from build123d import *

# Parameters (mm, degrees)
SKETCH_1_W             = 24
SKETCH_1_H             = 27
EXTRUDE_1_DEPTH        = 10
SKETCH_2_R             = 11
SKETCH_2_R_2           = 4.5
EXTRUDE_2_DEPTH        = 9
CUT_EXTRUDE_START      = -41
SKETCH_3_R             = 4.5
CUT_EXTRUDE_1_DEPTH    = 41
SKETCH_4_R             = 2.1
CUT_EXTRUDE_2_DEPTH    = 37.013519789
CHAMFER_1_SIZE         = 2
HOLE_WIZARD_M4_1_D     = 3.3
HOLE_WIZARD_M4_1_DEPTH = 11.5
HOLE_WIZARD_M4_1_TIP   = 0.991420021


with BuildPart() as part:
    # 草图1 → 凸台-拉伸1 (new body)
    with BuildSketch(Plane.XY):
        Rectangle(SKETCH_1_W, SKETCH_1_H)
    extrude(amount=EXTRUDE_1_DEPTH)

    # 草图2 → 凸台-拉伸2 (add)
    with BuildSketch(Plane.XY):
        Circle(SKETCH_2_R)
        Circle(SKETCH_2_R_2, mode=Mode.SUBTRACT)
    extrude(amount=-EXTRUDE_2_DEPTH)

    # 草图3 → 切除-拉伸1 (cut)
    with BuildSketch(Plane(origin=(0, 0, 0), x_dir=(-1, 0, 0), z_dir=(0, 0, -1)).offset(CUT_EXTRUDE_START)):
        with Locations(Location((0, 0, 0), (0, 0, 180))):
            Circle(SKETCH_3_R)
    extrude(amount=CUT_EXTRUDE_1_DEPTH, mode=Mode.SUBTRACT)

    # 草图4 → 切除-拉伸2 (cut)
    with BuildSketch(Plane(origin=(0, 13.5, 0), x_dir=(1, 0, 0), z_dir=(0, 1, 0))):
        with Locations(Location((-8, -5, 0), (0, 0, 270))):
            Circle(SKETCH_4_R)
        with Locations(Location((8, -5, 0), (0, 0, 270))):
            Circle(SKETCH_4_R)
    extrude(amount=-CUT_EXTRUDE_2_DEPTH, mode=Mode.SUBTRACT)

    # 倒角1
    chamfer_1_edges = [part.edges().sort_by_distance(p)[0] for p in [
        (12, 0, 10),
    ]]
    chamfer(chamfer_1_edges, length=CHAMFER_1_SIZE)

    # M4 螺纹孔1
    with Locations(Plane(origin=(11, 0, 0), x_dir=(0, 0, -1), z_dir=(1, 0, 0))):
        with Locations((3, 0)):
            Hole(HOLE_WIZARD_M4_1_D / 2, depth=HOLE_WIZARD_M4_1_DEPTH)
            with Locations((0, 0, -(HOLE_WIZARD_M4_1_DEPTH + HOLE_WIZARD_M4_1_TIP / 2))):  # 118° drill point
                Cone(0, HOLE_WIZARD_M4_1_D / 2, HOLE_WIZARD_M4_1_TIP, mode=Mode.SUBTRACT)


solid = part.part
Source: CAD feature listing. Evaluate the final solid. Frame: model axes, mm. A direction names the side the tool comes from. Round coordinates to 2 decimals unless told otherwise and drop trailing zeros. Loops run counter-clockwise (first coordinate to the right, second up) from the corner with the lowest first, then second, coordinate; pieces in that order, holes last.
Q1. Section D-D, the plane x = 8. Return loops of the section in (y, z).
Q2. Section C-C, the plane y = 1. Return loops of the section in (x, z).
Q3. Section B-B, the plane x = 0. Return loops of the section in (y, z), plus the area to 3 significant figures.
Q4. Ray query, line 1 (X direction, y = 6, z = 5); line 2 (Z direction, x = 7.5, y = -0.5); line 3 (Z direction, x = 7, y = 0). Return the intervals inside material, ascending.
Q5. First-contact query: P1, Ø3, axis at x = -7.5, z = -7, coming from the -Y side; P2, Ø5.5, axis at y = 0, z = -3, coming from the -X side; P3, Ø4, axis at x = 1.5, z = -5, coming from the +Y side; P4, Ø4, axis at x = -8, z = 5, coming from the -Y side. Flat tips, straight axial feed; report the tip coordinate or a pass-through.
Q6. Section A-A, the plane z = 5. Return loops of the section in (x, y).
Q7. Mould query, pull axis X, two halves, no side actions, for faces 1 (the face through (0, 13.5, 5)), 2 (the face through (11, 0, 9)), 3 (the face through (10.082, 0.189, 4.727)). Classes: pulls with the +X half, pulls with the -X half, needs draft (parallel to the pull), parting line crosses it, or undercut.
Q8. Access query for faces 4 (the face through (-4, 3, 10)), 5 (the face through (7.546, 0.496, -1.426)), 6 (the face through (-11, -3, 0)). Directions: +Z, -Z, +X, -X, +Y, -Y. A direction counts if a zero-diameter tool reaches every point of the face in a straight line with its end or side. Return the directions, or none.
Solutions:
1. outline: (-13.5, 0) - (-7.55, 0) - (-7.55, -9) - (7.55, -9) - (7.55, 0) - (13.5, 0) - (13.5, 2.9) - (-13.5, 2.9) - close; (-13.5, 7.1) - (13.5, 7.1) - (13.5, 10) - (-13.5, 10) - close; hole circle Ø3.3 at (0, -3)
2. outline: (-12, 0) - (-10.95, 0) - (-10.95, -9) - (-4.39, -9) - (-4.39, 10) - (-12, 10) - close; (4.39, -9) - (10.95, -9) - (10.95, -4.31) - (4.39, -4.31) - close; (4.39, -1.69) - (10.95, -1.69) - (10.95, 0) - (12, 0) - (12, 8) - (10, 10) - (4.39, 10) - close; hole circle Ø4.2 at (-8, 5); hole circle Ø4.2 at (8, 5)
3. outline: (-13.5, 0) - (-11, 0) - (-11, -9) - (-4.5, -9) - (-4.5, 10) - (-13.5, 10) - close; (4.5, -9) - (11, -9) - (11, 0) - (13.5, 0) - (13.5, 10) - (4.5, 10) - close
3. area: 297 mm2
4. line 1: x = -12 to -10.1, -5.9 to 5.9, 10.1 to 12
4. line 2: z = -9 to -4.57, -1.43 to 2.96, 7.04 to 10
4. line 3: z = -9 to -4.65, -1.35 to 3.15, 6.85 to 10
5. P1: stops at y = -9.22
5. P2: stops at x = -11
5. P3: stops at y = 11
5. P4: passes through
6. outline: (-12, -13.5) - (-10.1, -13.5) - (-10.1, 13.5) - (-12, 13.5) - close; (-5.9, -13.5) - (5.9, -13.5) - (5.9, 13.5) - (-5.9, 13.5) - close; (10.1, -13.5) - (12, -13.5) - (12, 13.5) - (10.1, 13.5) - close; hole circle Ø9 at (0, 0)
7. face 1: needs draft
7. face 2: pulls with the +X half
7. face 3: undercut
8. face 4: +Z, +X, -X, +Y, -Y
8. face 5: +X
8. face 6: -Z
